Job drawing, mm, ordinate dimensions from the low corner. One solid piece. Give positions to 0.01 mm unless a question says otherwise; leave off trailing zeros. Write each loop counter-clockwise with the first axis right and the second up, starting at its lowest first coordinate (ties: lowest second). Pieces come first, ordered by that corner, then holes. Notation, with made-up numbers: M 34.5,7.5 L 76.5,7.5 A24 ccw 76.5,39.5 Z; hole C 72.5,11.25 d2. An arc over 180 degrees is marked long. Answer as CSV lines item,"result". Start each with the question number.
1) Slice it at C-C, the plane x = 146. Give the cut face in (y, z), plus the area to 3 significant figures.
2) Pin check, flat tips, straight feed: pin 1 Ø3 at (y, z) = (1, 234.5) entering from -X; pin 2 Ø3 at (y, z) = (2.5, 109.5) entering from +X; pin 3 Ø1 at (y, z) = (4.5, 171) entering from +X (1 decimal). Stop position of each tip, or through.
3) Slice it at A-A, the plane y = 1. Give the cut face in (x, z).
4) Wall check: line 1 along X through (y, z) = (5, 210); line 2 along X through (y, z) = (4, 41.5) (1 decimal); line 3 along Z through (x, y) = (236.5, 5.5). Give the ranges that are in metal, low to high. Write a range as from..to.
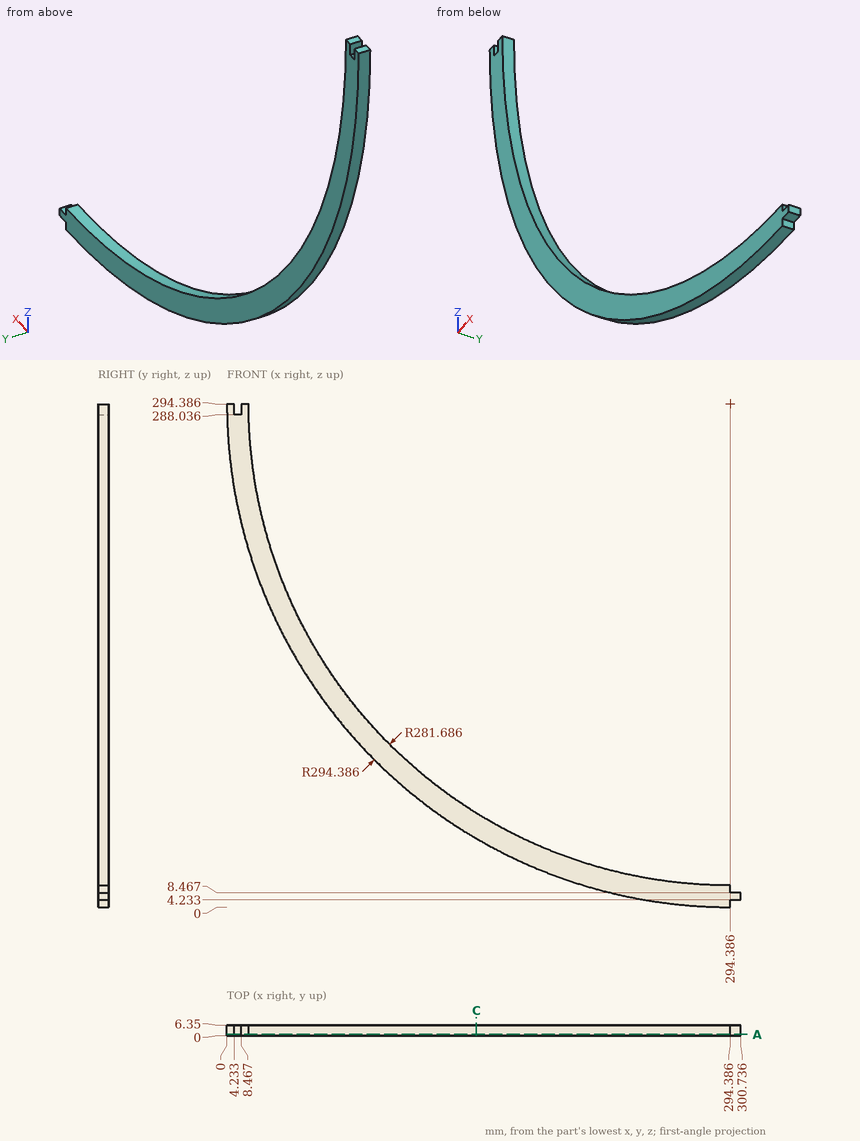
Found:
1,outline,"M 0,40.13 L 6.35,40.13 L 6.35,54.95 L 0,54.95 Z"
1,area,"94.1 mm²"
2,pin 1,"x = 5.85"
2,pin 2,"x = 83.18"
2,pin 3,"x = 41.4"
3,outline,"M 0,294.39 A294.39 ccw 294.39,0 L 294.39,4.23 L 300.74,4.23 L 300.74,8.47 L 294.39,8.47 L 294.39,12.7 A281.69 cw 12.7,294.39 L 8.47,294.39 L 8.47,288.04 L 4.23,288.04 L 4.23,294.39 Z"
4,line 1,"12.35..25.64"
4,line 2,"143.7..170.3"
4,line 3,"5.75..18.71"
